Autodesk Inventor part; units mm, degrees
ref_plane "pin_to_nut_XY" through (39.7, 0, 0) normal (1, 0, 0) x (0, 0, -1)
ref_plane "pin_to_nut_YZ" through (39.7, 0, 0) normal (0, 0, -1) x (0, 1, 0)
ref_plane "pin_to_nut_ZX" through (39.7, 0, 0) normal (0, 1, 0) x (1, 0, 0)
sketch "Sketch_1" plane through (0, 0, 0) normal (0, 0, 1) x (1, 0, 0)
  line L0 (44, 0) -> (-5, 0)
  line L1 (-2.2783, 0) -> (-3, 1.25)
  line L2 (-3, 1.25) -> (-5, 1.25)
  line L3 (-5, 1.25) -> (-5, 4)
  line L4 (-5, 4) -> (-4.5, 4.5)
  line L5 (-4.5, 4.5) -> (0, 4.5)
  line L6 (0, 4.5) -> (0, 2.45)
  line L7 (0, 2.45) -> (1.5, 2.45)
  line L8 (1.5, 2.45) -> (1.5, 2.5)
  line L9 (1.5, 2.5) -> (38, 2.5)
  line L10 (38, 2.5) -> (38, 1.85)
  arc A0 (38, 1.85) -> (38.3, 1.55) centre (38.3, 1.85) ccw
  line L11 (38.3, 1.55) -> (38.9, 1.55)
  arc A1 (38.9, 1.55) -> (39.2, 1.85) centre (38.9, 1.85) ccw
  line L12 (39.2, 1.85) -> (39.2, 2)
  line L13 (39.2, 2) -> (43.5705, 2)
  line L14 (43.5705, 2) -> (44, 1.5705)
  line L15 (44, 1.5705) -> (44, 0)
  line L16 (44, 0) -> (-2.2783, 0)
revolve "Revolution1" add sketch "Sketch_1" angle 360 about axis through (44, 0, 0) along (1, 0, 0)
thread "Thread1"
sketch "Sketch_2" plane through (-5, 0, 0) normal (1, 0, 0) x (0, 0, -1)
  line L0 (-1.25, -0.7217) -> (0, -1.4434)
  line L1 (0, -1.4434) -> (1.25, -0.7217)
  line L2 (1.25, -0.7217) -> (1.25, 0.7217)
  line L3 (1.25, 0.7217) -> (0, 1.4434)
  line L4 (0, 1.4434) -> (-1.25, 0.7217)
  line L5 (-1.25, 0.7217) -> (-1.25, -0.7217)
extrude "Extrusion1" cut sketch "Sketch_2" along normal blind 2
ref_plane "pin_to_nut_XY" through (39.7, 0, 0) normal (1, 0, 0) x (0, 0, -1)
ref_plane "pin_to_nut_YZ" through (39.7, 0, 0) normal (0, 0, -1) x (0, 1, 0)
ref_plane "pin_to_nut_ZX" through (39.7, 0, 0) normal (0, 1, 0) x (1, 0, 0)
properties part number "SCLBRU5-38.0_D"
Work out the finished part from the listing and answer in its coordinate system (mm). A direction names the side the tool comes from. Give positions to 0.01 mm unless a question says otherwise; leave off trailing zeros. Order: outer loops, then holes, each group sorted by start corner. A loop starts at its lowest first (then second) coordinate and runs counter-clockwise, first axis right, second up. Notation, with made-up numbers: (-0.75, 54) - (5.25, 54) arc R15 ccw to (5.25, 60) - close; hole circle Ø3 at (41, -22). An arc over 180 degrees is marked (long way). One line per item, written item: value. Start each with the question number.
1. Consider line 1 (X direction, y = -2.75, z = 2.5); line 2 (Y direction, x = 7, z = 0.5); line 3 (X direction, y = -1.25, z = 1). Determine where each line is inside the solid, lowest interval first.
2. For a pull along Z with two mould halves and no side action, classify faces 1 (the face through (-2.22, -0.59, 4.46)), 2 (the face through (-4.014, -1.088, -0.616)), 3 (the face through (44, 0, 0)) as released by +Z, released by -Z, zero draft, split by the parting line, or undercut.
3. Each of these flat-tipped pins is pushed along its axis until it touches: pin 1 Ø4 at (x, z) = (13.5, 1.5) entering from -Y; pin 2 Ø3 at (y, z) = (3, 0) entering from +X; pin 3 Ø1 at (x, y) = (23.5, -2) entering from +Z; pin 4 Ø0.7 at (x, y) = (-4, 0.5) entering from -Z. Where does it stop, or does it pass through?
4. Section A-A, the plane x = 40.5 is taken. Write down the section's boundary in (y, z), then the cut area to 3 significant figures.
5. Section B-B, the plane x = 18.5 is taken. Write down the section's boundary in (y, z).
6. Which of the six approach directions +Z, -Z, +X, -X, +Y, -Y give full straight-line access (tool end or side, diameter ignored) to faces 4 (the face through (-4.01, 1.08, -0.63)), 5 (the face through (41, 0, -2)), 6 (the face through (38, -2, 1))?
Filled sheet:
1. line 1: -5 to 0
1. line 2: -2.45 to 2.45
1. line 3: -5 to 38.13, 39.07 to 43.97
2. face 1: split by the parting line
2. face 2: undercut
2. face 3: zero draft
3. pin 1: y = -2.5
3. pin 2: x = 44
3. pin 3: z = 2
3. pin 4: z = -4.5
4. outline: circle Ø4 at (0, 0)
4. area: 12.6 mm²
5. outline: circle Ø5 at (0, 0)
6. face 4: -X
6. face 5: +X
6. face 6: none
